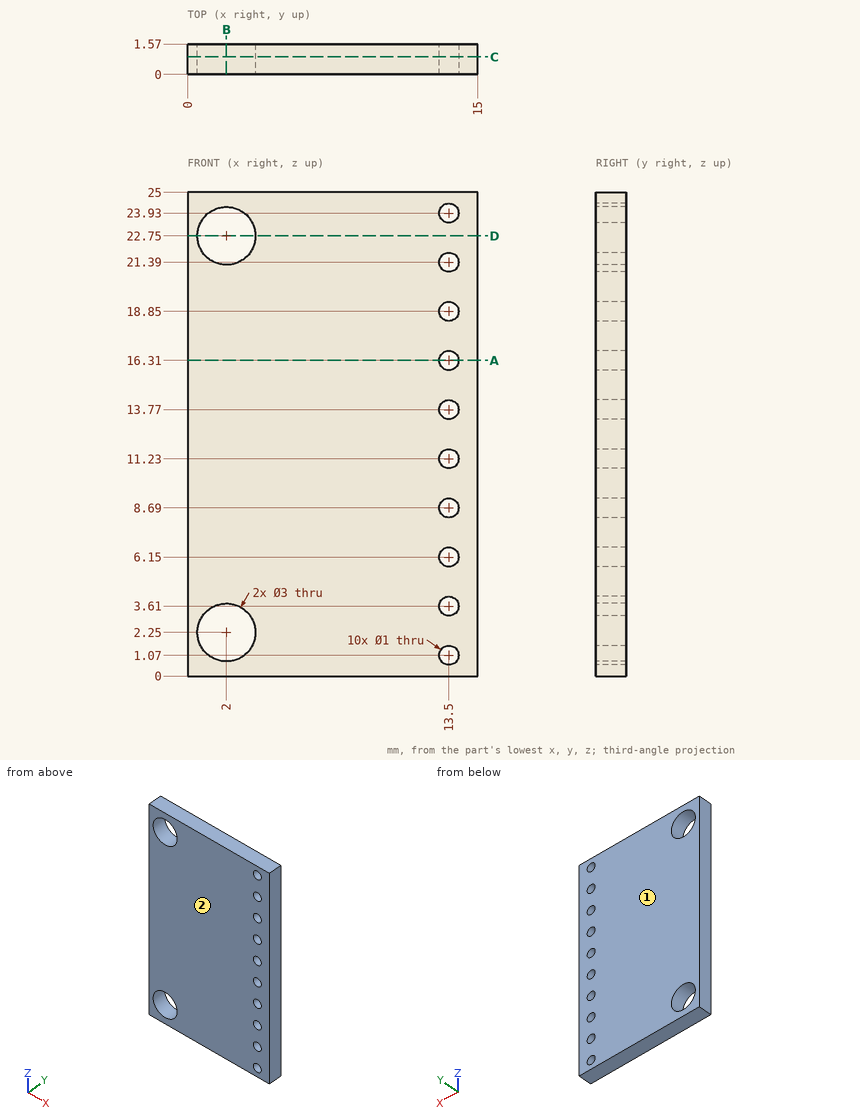
Input: dimensioned drawing with shaded views. Units: mm. Origin: part minimum x, y, z. Coordinates: 2 decimals unless noted, no trailing zeros. Loops run counter-clockwise (first coordinate to the right, second up) from the corner with the lowest first, then second, coordinate; pieces in that order, holes last. Notation, with made-up numbers: (22.25, 2) - (59.25, 2) arc R36 cw to (59.25, 36) - close; hole circle Ø9 at (72, 9). An arc over 180 degrees is marked (long way). One line per question, with ' | ' between items. Start each with the question number.
(1) Cut plane C-C on y = 0.9. Count the separate pieces of the cut face and the enclosed holes in it, and give its area (3 significant figures).
(2) Cut plane B-B on x = 2. Output: boundary loops of the cut face in (y, z), and give its area (3 significant figures).
(3) First-contact query: pin 1 (3 mm diameter, centred on x = 4, z = 16, fed in from -Y). Flat tip, straight axial feed; report the tip coordinate or a pass-through.
(4) Cut plane A-A on z = 16.31. Output: boundary loops of the cut face in (x, y), and give its area (3 significant figures).
(5) Draft query along Y for the marked faces 1 and 2. Return one class per face: +Y half, -Y half, draft (parallel to the pull), parting line (faces both ways), or undercut.
(6) Ray query, L1, parallel to Z at x = 1, y = 0.6; L2, parallel to Z at x = 3.25, y = 0.4; L3, parallel to X at y = 1.1, z = 8.75. Return the intervals inside material, ascending. Write a range as from..to.
(7) Cut plane D-D on z = 22.75. Output: boundary loops of the cut face in (x, y).
Here are the results:
1) separate pieces: 1 | enclosed holes: 12 | area: 353 mm²
2) outline: (0, 0) - (1.57, 0) - (1.57, 0.75) - (0, 0.75) - close; (0, 3.75) - (1.57, 3.75) - (1.57, 21.25) - (0, 21.25) - close; (0, 24.25) - (1.57, 24.25) - (1.57, 25) - (0, 25) - close | area: 29.8 mm²
3) pin 1: y = 0
4) outline: (0, 0) - (13, 0) - (13, 1.57) - (0, 1.57) - close; (14, 0) - (15, 0) - (15, 1.57) - (14, 1.57) - close | area: 22.0 mm²
5) face 1: +Y half | face 2: -Y half
6) L1: 0..1.13, 3.37..21.63, 23.87..25 | L2: 0..1.42, 3.08..21.92, 23.58..25 | L3: 0..13, 14..15
7) outline: (0, 0) - (0.5, 0) - (0.5, 1.57) - (0, 1.57) - close; (3.5, 0) - (15, 0) - (15, 1.57) - (3.5, 1.57) - close
